The listing builds one solid part. Answer for the finished solid, in the listing's coordinates (mm). Face numbers are marked on the shaded views. A direction names the side the tool comes from. Give positions to 0.01 mm unless a question says otherwise; leave off trailing zeros. Loops run counter-clockwise (first coordinate to the right, second up) from the corner with the lowest first, then second, coordinate; pieces in that order, holes last.
Item 1: Consider line 1 along X through (y, z) = (215.75, 16.5); line 2 along Z through (x, y) = (24.5, 233.75); line 3 along Z through (x, y) = (12.5, 213). Determine where each line is inside the solid, lowest interval first.
Item 2: The mould has two halves that part along X. Classify the marked faces 1, 2 and 3: pulls with the +X half, pulls with the -X half, needs draft (parallel to the pull), parting line crosses it, or undercut.
Item 3: Each of these flat-tipped pins is pushed along its axis until it touches: pin 1 Ø1.5 at (y, z) = (218.5, 20) entering from -X; pin 2 Ø3 at (x, z) = (22, 8) entering from +Y; pin 3 Ø4 at (y, z) = (227.5, 15) entering from +X; pin 4 Ø2.5 at (x, y) = (22.67, 216.92) entering from -Z. Where does it stop, or does it pass through?
Item 4: Section A-A, the plane y = 224 is taken. Give the vertices of the cut face in (x, z).
Item 5: Section C-C, the plane z = 27 is taken. Give the vertices of the cut face in (x, y).
Item 6: A tool of negligible diameter and unlimited length cuts with its end or side. For the marked faces 4, 5, 6, 7 and 8, from which of +Z, -Z, +X, -X, +Y, -Y can it reach the whole face along a straight path? Write none if from no direction.
Item 7: Section D-D, the plane y = 230.5 is taken. Give the number of separate pieces and of enclosed holes in the cut face, and give its area (3 significant figures).
Item 8: Section B-B, the plane x = 19 is taken. Give the vertices of the cut face in (y, z), and give its area (3 significant figures).
from build123d import *

# Parameters (mm, degrees)
SKETCH1_W           = 35
SKETCH1_H           = 25
SKETCH1_R           = 1.7
BOSS_EXTRUDE1_DEPTH = 5
BOSS_EXTRUDE2_DEPTH = 25
SKETCH4_R           = 1.7
CUT_EXTRUDE1_DEPTH  = 5
SKETCH5_R           = 3
SKETCH5_R_2         = 1.7
CUT_EXTRUDE3_DEPTH  = 3
BOSS_EXTRUDE3_DEPTH = 2
BOSS_EXTRUDE4_DEPTH = 1.5


with BuildPart() as part:
    # Sketch1 → Boss-Extrude1 (new body)
    with BuildSketch(Plane.XY):
        with Locations((10.173766162, 223.42362241)):
            Rectangle(SKETCH1_W, SKETCH1_H)
        with Locations((22.673766162, 216.923622409)):
            Circle(SKETCH1_R, mode=Mode.SUBTRACT)
        with Locations((22.673766162, 229.923622409)):
            Circle(SKETCH1_R, mode=Mode.SUBTRACT)
        with Locations((-2.326233838, 229.923622409)):
            Circle(SKETCH1_R, mode=Mode.SUBTRACT)
        with Locations((-2.326233838, 216.923622409)):
            Circle(SKETCH1_R, mode=Mode.SUBTRACT)
    extrude(amount=BOSS_EXTRUDE1_DEPTH)

    # Sketch3 → Boss-Extrude2 (add)
    with BuildSketch(Plane.XZ.offset(-210.92362241)):
        with BuildLine():
            Line((17.673766162, 28), (2.673766162, 28))
            Line((2.673766162, 28), (2.673766162, 16.5))
            Line((2.673766162, 16.5), (6.073766162, 16.5))
            ThreePointArc((6.073766162, 16.5), (10.173766162, 20.6), (14.273766162, 16.5))
            Line((14.273766162, 16.5), (17.673766162, 16.5))
            Line((17.673766162, 16.5), (17.673766162, 28))
        make_face()
        with BuildLine():
            Line((6.073766162, 16.5), (2.673766162, 16.5))
            Line((2.673766162, 16.5), (2.673766162, 5))
            Line((2.673766162, 5), (17.673766162, 5))
            Line((17.673766162, 5), (17.673766162, 16.5))
            Line((17.673766162, 16.5), (14.273766162, 16.5))
            ThreePointArc((14.273766162, 16.5), (10.173766162, 12.4), (6.073766162, 16.5))
        make_face()
        Polygon((27.673766162, 33), (-7.326233838, 33), (-7.326233838, 28), (2.673766162, 28), (17.673766162, 28), (27.673766162, 28), align=None)
    extrude(amount=-BOSS_EXTRUDE2_DEPTH)

    # Sketch4 → Cut-Extrude1 (cut)
    with BuildSketch(Plane(origin=(0, 0, 28), x_dir=(-1, 0, 0), z_dir=(0, 0, -1))):
        with Locations(Location((-22.673766162, 229.923622409, 0), (0, 0, 180))):
            Circle(SKETCH4_R)
        with Locations(Location((-22.673766162, 216.923622409, 0), (0, 0, 180))):
            Circle(SKETCH4_R)
        with Locations(Location((2.326233838, 229.923622409, 0), (0, 0, 180))):
            Circle(SKETCH4_R)
        with Locations(Location((2.326233838, 216.923622409, 0), (0, 0, 180))):
            Circle(SKETCH4_R)
    extrude(amount=-CUT_EXTRUDE1_DEPTH, mode=Mode.SUBTRACT)

    # Sketch5 → Cut-Extrude3 (cut)
    # profile 1 of 4: a face of its own
    with BuildSketch(Plane(origin=(0, 0, 28), x_dir=(-1, 0, 0), z_dir=(0, 0, -1))):
        with Locations((2.326233838, 216.923622409)):
            Circle(SKETCH5_R)
        with Locations((2.326233838, 216.923622409)):
            Circle(SKETCH5_R_2, mode=Mode.SUBTRACT)
    # profile 2 of 4: a face of its own
    with BuildSketch(Plane(origin=(0, 0, 28), x_dir=(-1, 0, 0), z_dir=(0, 0, -1))):
        with Locations((2.326233838, 229.923622409)):
            Circle(SKETCH5_R)
        with Locations((2.326233838, 229.923622409)):
            Circle(SKETCH5_R_2, mode=Mode.SUBTRACT)
    # profile 3 of 4: a face of its own
    with BuildSketch(Plane(origin=(0, 0, 28), x_dir=(-1, 0, 0), z_dir=(0, 0, -1))):
        with Locations((-22.673766162, 216.923622409)):
            Circle(SKETCH5_R)
        with Locations((-22.673766162, 216.923622409)):
            Circle(SKETCH5_R_2, mode=Mode.SUBTRACT)
    # profile 4 of 4: a face of its own
    with BuildSketch(Plane(origin=(0, 0, 28), x_dir=(-1, 0, 0), z_dir=(0, 0, -1))):
        with Locations((-22.673766162, 229.923622409)):
            Circle(SKETCH5_R)
        with Locations((-22.673766162, 229.923622409)):
            Circle(SKETCH5_R_2, mode=Mode.SUBTRACT)
    extrude(amount=-CUT_EXTRUDE3_DEPTH, mode=Mode.SUBTRACT)

    # Sketch6 → Boss-Extrude3 (add)
    with BuildSketch(Plane.XZ.offset(-210.92362241)):
        Polygon((-7.326233838, 0), (27.673766162, 0), (27.673766162, 5), (17.673766162, 5), (17.673766162, 28), (27.673766162, 28), (27.673766162, 33), (-7.326233838, 33), (-7.326233838, 28), (2.673766162, 28), (2.673766162, 5), (-7.326233838, 5), align=None)
    extrude(amount=-BOSS_EXTRUDE3_DEPTH)

    # Sketch7 → Boss-Extrude4 (add, symmetric)
    with BuildSketch(Plane(origin=(0, 223.42362241, 0), x_dir=(1, 0, 0), z_dir=(0, 1, 0))):
        Polygon((17.673766162, -28), (27.673766162, -28), (17.673766162, -18), align=None)
        Polygon((17.673766162, -5), (17.673766162, -15), (27.673766162, -5), align=None)
        Polygon((-7.326233838, -5), (2.673766162, -15), (2.673766162, -5), align=None)
        Polygon((2.673766162, -18), (-7.326233838, -28), (2.673766162, -28), align=None)
    extrude(amount=BOSS_EXTRUDE4_DEPTH, both=True)


solid = part.part
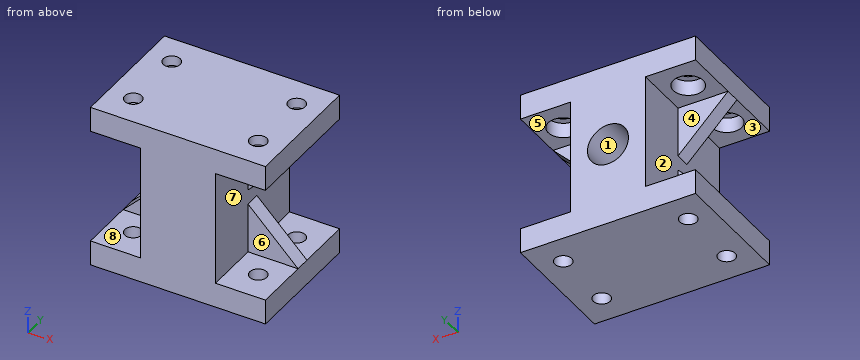
Worked answers:
1. line 1: x = 2.67 to 6.07, 14.27 to 17.67
1. line 2: z = 0 to 5, 28 to 33
1. line 3: z = 0 to 13.12, 19.88 to 33
2. face 1: undercut
2. face 2: pulls with the -X half
2. face 3: needs draft
3. pin 1: stops at x = 2.67
3. pin 2: stops at y = 224.92
3. pin 3: stops at x = 17.67
3. pin 4: passes through
4. outline: (-7.33, 0) - (27.67, 0) - (27.67, 5) - (17.67, 15) - (17.67, 18) - (27.67, 28) - (27.67, 33) - (-7.33, 33) - (-7.33, 28) - (2.67, 18) - (2.67, 15) - (-7.33, 5) - close; hole circle Ø8.2 at (10.17, 16.5)
5. outline: (-6.33, 221.92) - (2.67, 221.92) - (2.67, 210.92) - (17.67, 210.92) - (17.67, 221.92) - (26.67, 221.92) - (26.67, 224.92) - (17.67, 224.92) - (17.67, 235.92) - (2.67, 235.92) - (2.67, 224.92) - (-6.33, 224.92) - close
6. face 4: -X, +Y
6. face 5: +X, +Y
6. face 6: +X, -Y
6. face 7: +X
6. face 8: -X, -Y
7. separate pieces: 5
7. enclosed holes: 1
7. area: 562 mm2
8. outline: (210.92, 0) - (235.92, 0) - (235.92, 5) - (224.92, 5) - (224.92, 13.67) - (221.92, 13.67) - (221.92, 5) - (210.92, 5) - close; (210.92, 28) - (221.92, 28) - (221.92, 19.33) - (224.92, 19.33) - (224.92, 28) - (235.92, 28) - (235.92, 33) - (210.92, 33) - close
8. area: 302 mm2
